Answer from the drawing. Dimensions are ordinates in mm from the lowest x, y and z of the part. A direction names the side the tool comes from. Give positions to 0.01 mm unless a question says otherwise; leave off trailing zeros. Loops run counter-clockwise (first coordinate to the right, second up) from the corner with the lowest first, then second, coordinate; pieces in that order, holes last. Notation, with made-up numbers: (68, -32) - (74, -32) arc R15 cw to (74, -16) - close; hole circle Ø6 at (-35.75, -23). An arc over 180 degrees is marked (long way). One line per item, written item: value.
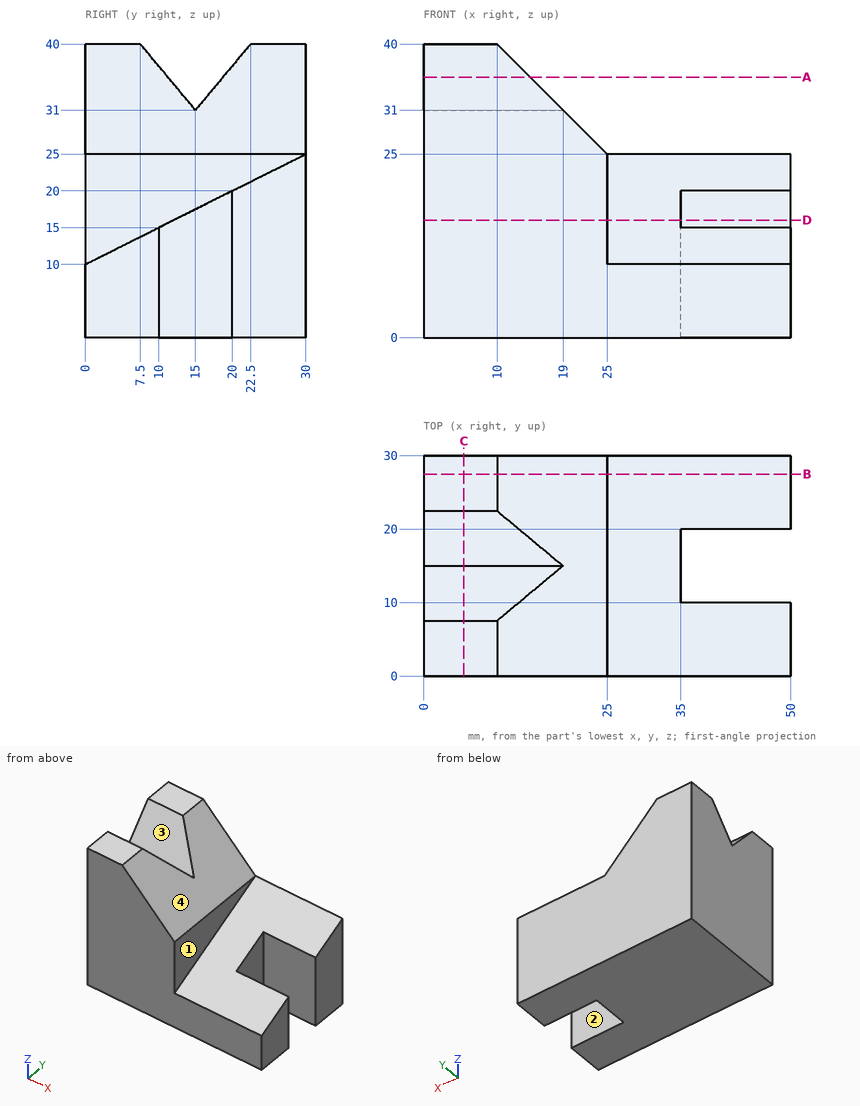
1. Section B-B (y = 27.5) is taken. Write down the section's boundary in (x, z).
Output:
outline: (0, 0) - (50, 0) - (50, 23.75) - (25, 23.75) - (25, 25) - (10, 40) - (0, 40) - close
2. Section D-D (z = 16) is taken. Write down the section's boundary in (x, y), and give its area (3 significant figures).
Output:
outline: (0, 0) - (25, 0) - (25, 12) - (35, 12) - (35, 20) - (50, 20) - (50, 30) - (0, 30) - close
area: 1,080 mm²
3. Section C-C (x = 5.5) is taken. Write down the section's boundary in (y, z), and give its area (3 significant figures).
Output:
outline: (0, 0) - (30, 0) - (30, 40) - (22.5, 40) - (15, 31) - (7.5, 40) - (0, 40) - close
area: 1,130 mm²
4. For the marked faces 1, 2, 3 and 4, determine the directions among +Z, -Z, +X, -X, +Y, -Y from which every point of the face is accessible in a straight line to the end or side of a thin tool.
Output:
face 1: +Z, +X, -Y
face 2: +Z, -Z, +X
face 3: +Z, +X, -X
face 4: +Z, +X, +Y, -Y
5. Flat-ended cylindrical pins translate along their axes: pin 1 Ø5 at (x, y) = (19.5, 26) entering from +Z; pin 2 Ø6 at (y, z) = (21, 21) entering from -X; pin 3 Ø1.5 at (x, y) = (14.5, 23.5) entering from +Z. Find the tip coordinate at first contact, or state that the pin passes through.
Output:
pin 1: stops at z = 33
pin 2: stops at x = 0
pin 3: stops at z = 36.25
6. Find the intervals of material crossed by line 1 along X through (y, z) = (12.25, 11.5); line 2 along Y through (x, z) = (42, 19.5); line 3 along X through (y, z) = (8.5, 22), in increasing order.
Output:
line 1: x = 0 to 35
line 2: y = 20 to 30
line 3: x = 0 to 25
7. Section A-A (z = 35.5) is taken. Write down the section's boundary in (x, y).
Output:
outline: (0, 0) - (14.5, 0) - (14.5, 11.25) - (0, 11.25) - close; (0, 18.75) - (14.5, 18.75) - (14.5, 30) - (0, 30) - close
